Could you check a few things on this model? Use its own coordinates, in mm. A direction names the side the tool comes from. Round coordinates to 2 decimals unless told otherwise and drop trailing zeros. Loops run counter-clockwise (first coordinate to the right, second up) from the corner with the lowest first, then second, coordinate; pieces in that order, holes last. Notation, with made-up numbers: (-33, 71) -> (18, 71) arc R21 ccw to (18, 79) -> close; hole circle Ø5 at (66, -14.5). An arc over 180 degrees is marked (long way). One line per item, written item: value.
```python
from build123d import *

# Parameters (mm, degrees)
F0_W     = 1036
F0_H     = 2236
F0_W_2   = 1000
F0_H_2   = 2200
F1_DEPTH = 1200
F2_W     = 1036
F2_H     = 2236
F3_DEPTH = 18
F4_W     = 836
F4_H     = 1068
F5_DEPTH = 18


with BuildPart() as f1:
    # F0 (on Top) → F1 (new body)
    with BuildSketch(Plane.XY):
        with Locations((518, 1118)):
            Rectangle(F0_W, F0_H)
        with Locations((518, 1118)):
            Rectangle(F0_W_2, F0_H_2, mode=Mode.SUBTRACT)
    extrude(amount=F1_DEPTH)

    # F2 (on face) → F3 (join)
    with BuildSketch(Plane(origin=(0, 0, 0), x_dir=(1, 0, 0), z_dir=(0, 0, -1))):
        with Locations((518, -1118)):
            Rectangle(F2_W, F2_H)
    extrude(amount=F3_DEPTH)

    # F4 (on face) → F5 (cut)
    with BuildSketch(Plane.XZ):
        with Locations((518, 516)):
            Rectangle(F4_W, F4_H)
    extrude(amount=-F5_DEPTH, mode=Mode.SUBTRACT)


solid = f1.part
```
Item 1: Will these pins go through, and if not, where does the flat tip stop? pin 1 Ø10 at (x, y) = (456.5, 665.5) entering from +Z; pin 2 Ø9 at (x, y) = (631.5, 9.5) entering from -Z; pin 3 Ø12 at (x, z) = (488, 299.5) entering from -Y.
Output:
pin 1: stops at z = 0
pin 2: stops at z = 1050
pin 3: stops at y = 2218
Item 2: If we section it at A-A on x = 560: List the corners of the cut face in (y, z) for me, plus the area to 3 significant figures.
Output:
outline: (0, 1050) -> (18, 1050) -> (18, 1200) -> (0, 1200) -> close; (18, -18) -> (2236, -18) -> (2236, 1200) -> (2218, 1200) -> (2218, 0) -> (18, 0) -> close
area: 64,200 mm²
Item 3: I need wall thicknesses on line 1 (X direction, y = 2030, z = 573.5); line 2 (Y direction, x = 983.5, z = 1022); line 3 (Z direction, x = 842.5, y = 552.5). Which ranges of each line are inside material? Lowest first, please. Write a range as from..to.
Output:
line 1: x = 0..18, 1018..1036
line 2: y = 0..18, 2218..2236
line 3: z = -18..0
Item 4: For faces 1 (the face through (18, 1103, 592)), 2 (the face through (0, 1134, 600)), which set-ups out of +Z, -Z, +X, -X, +Y, -Y let a thin tool reach every point of the face, with its end or its side?
Output:
face 1: +Z
face 2: +Z, -Z, -X, +Y, -Y
Item 5: If we mould it in two halves opening along X, with no side actions, what happens to faces 3 (the face through (1036, 1134, 600)), 4 (the face through (511, 2236, 600)), 5 (the face through (553, 18, 1086))? For each: released by +X, released by -X, zero draft, split by the parting line, or undercut.
Output:
face 3: released by +X
face 4: zero draft
face 5: undercut
Item 6: If we section it at D-D on y = 911.5: List the corners of the cut face in (x, z) for me, plus the area to 3 significant figures.
Output:
outline: (0, -18) -> (1036, -18) -> (1036, 1200) -> (1018, 1200) -> (1018, 0) -> (18, 0) -> (18, 1200) -> (0, 1200) -> close
area: 61,800 mm²
Item 7: If we section it at B-B on z = 400.5: List the corners of the cut face in (x, y) for me, plus the area to 3 significant figures.
Output:
outline: (0, 0) -> (100, 0) -> (100, 18) -> (18, 18) -> (18, 2218) -> (1018, 2218) -> (1018, 18) -> (936, 18) -> (936, 0) -> (1036, 0) -> (1036, 2236) -> (0, 2236) -> close
area: 101,000 mm²
Item 8: If we section it at C-C on x = 965: List the corners of the cut face in (y, z) for me, plus the area to 3 significant figures.
Output:
outline: (0, -18) -> (2236, -18) -> (2236, 1200) -> (2218, 1200) -> (2218, 0) -> (18, 0) -> (18, 1200) -> (0, 1200) -> close
area: 83,400 mm²
